The listing builds one solid part. Answer for the finished solid, in the listing's coordinates (mm). A direction names the side the tool comes from. Coordinates: 2 decimals unless noted, no trailing zeros. Write each loop counter-clockwise with the first axis right and the second up, starting at its lowest first coordinate (ties: lowest second). Pieces come first, ordered by that corner, then holes. Notation, with made-up numbers: M -26.75,-11.75 L 21.25,-11.75 A20 ccw 21.25,3.25 Z; hole C 51,66 d6. An arc over 180 degrees is marked long. Put each result on its own line as item: value. Start each with the question number.
Autodesk Inventor part; units mm, degrees
ref_plane "YZ Plane" through (0, 0, 0) normal (1, 0, 0) x (0, 1, 0)
ref_plane "XZ Plane" through (0, 0, 0) normal (0, 1, 0) x (-1, 0, 0)
ref_plane "XY Plane" through (0, 0, 0) normal (0, 0, 1) x (1, 0, 0)
sketch "Sketch1" plane through (0, 0, 0) normal (0, 1, 0) x (-1, 0, 0)
  line L0 (0, 75) -> (0, -75) construction
  arc A0 (18.258988, 69.745538) -> (-18.258988, 69.745538) centre (0, 75) ccw
  line L1 (0, -196.504208) -> (0, 248.158352) construction
  line L2 (-25.341268, -40) -> (25.341268, -40)
  line L3 (25.341268, -40) -> (20, -23.743159)
  line L4 (20, -23.743159) -> (-20, -23.743159)
  line L5 (-20, -23.743159) -> (-25.341268, -40)
  circle A1 centre (12, -31.871075) radius 2
  circle A2 centre (-12, -31.871075) radius 2
  circle A3 centre (0, -31.871075) radius 2
  circle A4 centre (0, -75) radius 23.5
  circle A5 centre (170.873428, 25.827072) radius 158.808057
  circle A6 centre (-170.873428, 25.827072) radius 158.808057
  point P0 (0, 0)
  dimension "d0" = 150
  dimension "d1" = 75
  dimension "d22" = 38
  dimension "d33" = 47
  dimension "d34" = 4
  dimension "d35" = 71.8118
  dimension "d36" = 71.8118
  dimension "d37" = 16.25684
  dimension "d38" = 35
  dimension "d39" = 35
  dimension "d40" = 0
  dimension "d41" = 48.15025
  dimension "d42" = 0
  dimension "d43" = 48.15025
  dimension "d44" = 0
  dimension "d45" = 8.12893
  dimension "d46" = 10.13733
  dimension "d47" = 8.12893
  dimension "d48" = 21.53777
  dimension "d49" = 8.12893
  dimension "d50" = 32.93821
  dimension "d51" = 0
  dimension "d52" = 16.25684
  dimension "d53" = 38.00145
  dimension "d54" = 16.25684
extrude "Extrusion1" add sketch "Sketch1" along normal blind 10 contours A5 L4 A6 A0 | L3 L2 L5 L4 | A1 | A2
sketch "Sketch4" plane through (0, 10, 0) normal (0, 1, 0) x (1, 0, 0)
  circle A0 centre (3.680608, -72.875) radius 1.5
  circle A1 centre (0, -79.25) radius 1.5
  circle A2 centre (-3.680608, -72.875) radius 1.5
  arc A3 (5.450881, -75.044363) -> (2.76386, -79.69842) centre (10.238345, -80.911111) ccw
  arc A4 (5.450881, -75.044363) -> (2.687021, -70.257217) centre (3.680608, -72.875) ccw
  arc A5 (-2.687021, -70.257217) -> (2.687021, -70.257217) centre (0, -63.177778) ccw
  arc A6 (-2.687021, -70.257217) -> (-5.450881, -75.044363) centre (-3.680608, -72.875) ccw
  arc A7 (-2.76386, -79.69842) -> (-5.450881, -75.044363) centre (-10.238345, -80.911111) ccw
  arc A8 (-2.76386, -79.69842) -> (2.76386, -79.69842) centre (0, -79.25) ccw
  point P0 (0, 0)
extrude "Extrusion4" cut sketch "Sketch4" against normal through all contours A0 | A1 | A2
sketch "Sketch5" plane through (0, 10, 0) normal (0, 1, 0) x (1, 0, 0)
  circle A0 centre (-3.680608, -72.875) radius 1.5
  circle A1 centre (-3.680608, -72.875) radius 2.225
  circle A2 centre (0, -79.25) radius 1.5
  circle A3 centre (0, -79.25) radius 2.225
  circle A4 centre (3.680608, -72.875) radius 1.5
  circle A5 centre (3.680608, -72.875) radius 2.225
  point P0 (0, 0)
  dimension "d69" = 4.45
  dimension "d70" = 4.45
  dimension "d71" = 4.45
extrude "Extrusion5" cut sketch "Sketch5" against normal blind 6 contours A0 | A1 | A2 | A3 | A4 | A5
sketch "Sketch6" plane through (0, 0, 0) normal (0, -1, 0) x (1, 0, 0)
  circle A0 centre (0, 79.25) radius 1.5
  circle A1 centre (3.680608, 72.875) radius 1.5
  circle A2 centre (-3.680608, 72.875) radius 1.5
  point P0 (0, 0)
extrude "Extrusion6" add sketch "Sketch6" against normal up to surface (4 mm away)
sketch "Sketch7" plane through (0, 0, 0) normal (0, -1, 0) x (1, 0, 0)
  circle A0 centre (23.270461, -31.871075) radius 2
  circle A1 centre (-23.270461, -31.871075) radius 2
  circle A2 centre (0, -31.871075) radius 2
  line L0 (-32.726793, -40) -> (32.726793, -40)
  line L1 (-29.32798, -23.743159) -> (29.32798, -23.743159)
  line L2 (-25.341268, -40) -> (-20, -23.743159)
  line L3 (20, -23.743159) -> (25.341268, -40)
  line L4 (29.32798, -23.743159) -> (32.726793, -40)
  line L5 (-32.726793, -40) -> (-29.32798, -23.743159)
  point P0 (0, 0)
  point P1 (22.130539, -30.227731)
  point P2 (23.327313, -33.870267)
  point P3 (-23.327313, -33.870267)
  point P4 (-22.130539, -30.227731)
extrude "Extrusion7" add sketch "Sketch7" against normal up to surface (10 mm away) contours A0 L3 | A0 L3 L1 L4 L0 | L2 A1 L0 L5 L1 | L2 A1 | A1 L2 picked at (24.149861, -31.36133)
sketch "Sketch8" plane through (0, 10, 0) normal (0, 1, 0) x (1, 0, 0)
  arc A0 (-18.258988, -69.745538) -> (18.258988, -69.745538) centre (0, -75) ccw
  line L0 (0, -75) -> (0, -57.620328) construction
  line L1 (-29.32798, 23.743159) -> (-32.726793, 40)
  line L2 (-29.32798, 23.743159) -> (-18.322098, -28.899016)
  arc A1 (-18.553855, -70.906779) -> (-18.322098, -28.899016) centre (-116.205725, -49.363513) ccw
  arc A2 (-18.258988, -69.745538) -> (18.258988, -69.745538) centre (0, -75) ccw
  circle A3 centre (0, -75) radius 19
  arc A4 (-18.258988, -69.745538) -> (-20, 23.743159) centre (-170.873428, -25.827072) ccw
  line L3 (-20, 23.743159) -> (-29.32798, 23.743159)
  arc A5 (20, 23.743159) -> (18.258988, -69.745538) centre (170.873428, -25.827072) ccw
  line L4 (29.32798, 23.743159) -> (20, 23.743159)
  line L5 (29.32798, 23.743159) -> (18.322098, -28.899016)
  arc A6 (18.322098, -28.899016) -> (18.553855, -70.906779) centre (116.205725, -49.363513) ccw
  point P0 (0, 0)
  point P1 (18.553855, -70.906779)
  point P2 (-18.553855, -70.906779)
  dimension "d80" = 100
extrude "Extrusion8" add sketch "Sketch8" against normal blind 10 contours A0 A1 L2 L3 A4 | A5 L4 L5 A6 A0
sketch "Sketch11" plane through (0, 0, 0) normal (0, -1, 0) x (1, 0, 0)
  circle A0 centre (23.270461, -31.871075) radius 2
  circle A1 centre (-23.270461, -31.871075) radius 2
  point P0 (0, 0)
extrude "Extrusion11" cut sketch "Sketch11" against normal through all
chamfer "Chamfer1" distance 2 angle 45 5 edges at (-25.5244, 0, -5.5505) (-16.2072, 0, 49.9152) (0, 0, 94) (16.2072, 0, 49.9152) (25.5244, 0, -5.5505)
sketch "Sketch17" plane through (0, 10, 0) normal (0, 1, 0) x (1, 0, 0)
  line L0 (-83.121979, 82.295999) -> (15.75457, -64.379571)
  line L1 (-29.32798, 23.743159) -> (29.32798, 23.743159)
  circle A0 centre (-23.270461, 31.871075) radius 2
  circle A1 centre (23.270461, 31.871075) radius 2
  circle A2 centre (0, 31.871075) radius 2
  arc A3 (-18.553855, -70.906779) -> (18.553855, -70.906779) centre (0, -75) ccw
  arc A4 (18.322098, -28.899016) -> (18.553855, -70.906779) centre (116.205725, -49.363513) ccw
  line L2 (32.726793, 40) -> (18.322098, -28.899016)
  line L3 (-32.726793, 40) -> (32.726793, 40)
  line L4 (-32.726793, 40) -> (-18.322098, -28.899016)
  arc A5 (-18.553855, -70.906779) -> (-18.322098, -28.899016) centre (-116.205725, -49.363513) ccw
  circle A6 centre (-3.680608, -72.875) radius 2.225
  circle A7 centre (0, -79.25) radius 2.225
  circle A8 centre (3.680608, -72.875) radius 2.225
  line L5 (15.75457, -64.379571) -> (17.86641, -67.512319)
  line L6 (-32.726793, 40) -> (-18.322098, -28.899016)
  point P0 (0, 0)
  point P1 (-22.889065, -7.054783)
extrude "Extrusion16" add sketch "Sketch17" along normal blind 9 contours L4 L1 L2 A4 L5 L0
sketch "Sketch18" plane through (0, 19, 0) normal (0, 1, 0) x (1, 0, 0)
  circle A0 centre (13.844472, -83.053003) radius 1.5
  circle A1 centre (-8.053003, -88.844472) radius 1.5
  circle A2 centre (8.053003, -61.155528) radius 1.5
  circle A3 centre (-13.844472, -66.946997) radius 1.5
  circle A4 centre (57.038778, -59.914319) radius 1.5
  circle A5 centre (0, -75) radius 12.1825
  line L0 (54.737573, -51.213489) -> (22.535282, -59.730387)
  arc A6 (59.339984, -68.61515) -> (54.737573, -51.213489) centre (57.038778, -59.914319) ccw
  line L1 (27.137693, -77.132048) -> (59.339984, -68.61515)
  arc A7 (27.137693, -77.132048) -> (15.997897, -85.250234) centre (31.995793, -95.500468) ccw
  arc A8 (8.838591, -58.180983) -> (15.997897, -85.250234) centre (0, -75) ccw
  arc A9 (8.838591, -58.180983) -> (22.535282, -59.730387) centre (17.677181, -41.361967) ccw
  arc A10 (18.322098, -28.899016) -> (17.86641, -67.512319) centre (116.205725, -49.363513) ccw
  line L2 (18.322098, -28.899016) -> (29.32798, 23.743159)
  line L3 (29.32798, 23.743159) -> (-29.32798, 23.743159)
  line L4 (-29.32798, 23.743159) -> (-22.889065, -7.054783)
  line L5 (-22.889065, -7.054783) -> (17.86641, -67.512319)
  circle A11 centre (-19.580037, -5.657222) radius 3.525
  circle A12 centre (14.082222, -57.518268) radius 2.448572
  arc A13 (18.322098, -28.899016) -> (17.86641, -67.512319) centre (116.205725, -49.363513) ccw
  point P0 (0, 0)
  point P1 (-22.502925, -7.627592)
  point P2 (-23.030435, -6.378596)
  point P3 (16.523025, -57.323365)
  point P4 (12.051896, -58.886946)
  dimension "d117" = 7.05
extrude "Extrusion17" cut sketch "Sketch18" against normal up to surface (9 mm away) contours A10 L5 A9 | A9 A12 A10 | A9 L5 A12 | L5 L4 A11
sketch "Sketch19" plane through (0, 19, 0) normal (0, 1, 0) x (1, 0, 0)
  arc A0 (-23.030435, -6.378596) -> (-22.502925, -7.627592) centre (-19.580037, -5.657222) ccw
  circle A1 centre (-19.580037, -5.657222) radius 2.225
  circle A2 centre (12.769294, -53.644906) radius 3.525 construction
  line L0 (-22.502925, -7.627592) -> (12.051896, -58.886946)
  arc A3 (18.322098, -28.899016) -> (16.523025, -57.323365) centre (116.205725, -49.363513) ccw
  circle A4 centre (12.769294, -53.644906) radius 2.225
  point P0 (0, 0)
  dimension "d120" = 4.45
  dimension "d121" = 7.05
  dimension "d122" = 4.45
extrude "Extrusion18" cut sketch "Sketch19" against normal blind 9.5
sketch "Sketch20" plane through (0, 19, 0) normal (0, 1, 0) x (1, 0, 0)
  circle A0 centre (-19.580037, -5.657222) radius 2.225
  circle A1 centre (12.769294, -53.644906) radius 2.225
  arc A2 (-23.030435, -6.378596) -> (-22.502925, -7.627592) centre (-19.580037, -5.657222) ccw
  line L0 (-22.502925, -7.627592) -> (12.051896, -58.886946)
  arc A3 (12.051896, -58.886946) -> (16.523025, -57.323365) centre (14.082222, -57.518268) ccw
  arc A4 (18.322098, -28.899016) -> (16.523025, -57.323365) centre (116.205725, -49.363513) ccw
  line L1 (18.322098, -28.899016) -> (29.32798, 23.743159)
  line L2 (29.32798, 23.743159) -> (-29.32798, 23.743159)
  line L3 (-29.32798, 23.743159) -> (-23.030435, -6.378596)
  line L4 (-13.501752, -3.090072) -> (7.292792, -33.93714)
  arc A5 (8.533736, -26.852566) -> (7.292792, -33.93714) centre (116.205725, -49.363513) ccw
  line L5 (8.533736, -26.852566) -> (17.02107, 13.743159)
  line L6 (17.02107, 13.743159) -> (-17.02107, 13.743159)
  line L7 (-17.02107, 13.743159) -> (-13.501752, -3.090072)
  point P0 (0, 0)
  dimension "d125" = 10
extrude "Extrusion19" cut sketch "Sketch20" against normal through all contours L7 L6 L5 A5 L4
fillet "Fillet2" radius 5 4 edges at (-13.5018, 9.5, 3.0901) (7.2928, 9.5, 33.9371) (-17.0211, 9.5, -13.7432) (17.0211, 9.5, -13.7432)
sketch "Sketch21" plane through (0, 10, 0) normal (0, 1, 0) x (1, 0, 0)
  line L0 (12.051896, -58.886946) -> (-22.502925, -7.627592)
  arc A0 (-23.030435, -6.378596) -> (-22.502925, -7.627592) centre (-19.580037, -5.657222) ccw
  line L1 (-23.030435, -6.378596) -> (-18.322098, -28.899016)
  arc A1 (-18.553855, -70.906779) -> (-18.322098, -28.899016) centre (-116.205725, -49.363513) ccw
  arc A2 (-18.553855, -70.906779) -> (18.553855, -70.906779) centre (0, -75) ccw
  arc A3 (16.523025, -57.323365) -> (18.553855, -70.906779) centre (116.205725, -49.363513) ccw
  arc A4 (12.051896, -58.886946) -> (16.523025, -57.323365) centre (14.082222, -57.518268) ccw
  circle A5 centre (-3.680608, -72.875) radius 2.225
  circle A6 centre (0, -79.25) radius 2.225
  circle A7 centre (3.680608, -72.875) radius 2.225
  circle A8 centre (0, -75) radius 8.5 construction
  circle A9 centre (0, -75) radius 9.35
  point P0 (0, 0)
  dimension "d129" = 17
  dimension "d130" = 0.85
extrude "Extrusion20" cut sketch "Sketch21" against normal blind 0.2 contours A4 A3 A2 A1 L1 A0 L0
chamfer "Chamfer2" distance 0.2 angle 45 1 edges at (-9.35, 9.8, 75)
properties part number "motion_thigh_bot_3DPrint"
1) Straight lines are drawn through the part: probe 1 along X at (y, z) = (12.25, 4); probe 2 along Z at (x, y) = (0, 5.65) (3 decimals); probe 3 along Y at (x, z) = (6.5, 61.5). For each, find the intervals that lie inside material, in ascending order.
2) A cutting plane is placed at A-A on x = 24. Write down the section's boundary in (y, z).
3) A cutting plane is placed at C-C on z = -22.5. Write down the section's boundary in (x, y), then the cut area to 3 significant figures.
4) A cutting plane is placed at B-B on z = 0. Write down the section's boundary in (x, y), then the cut area to 3 significant figures.
5) For faces 4 (the face through (-16.21, 5.95, 50.21)), 5 (the face through (13, 19, 8)), 6 (the face through (-4, 4, 73)), 7 (the face through (0, 10, -35)), 8 (the face through (-6.325, 9.633, 13.736)), determine the directions among +Z, -Z, +X, -X, +Y, -Y from which every point of the face is accessible in a straight line to the end or side of a thin tool.
6) Given pin 1 Ø1 at (y, z) = (10, -19.5) entering from -X; pin 2 Ø8 at (x, z) = (9.5, 2) entering from +Y; pin 3 Ø4 at (x, z) = (12.77, 53.64) entering from +Y; pin 4 Ø8 at (x, y) = (-8.5, 15) entering from -Z, each flat-ended and moving along its own axis, determine where each tip first touches the part or whether it passes through.
7) Determine the mould class of faces 1 (the face through (0, 10, 75)), 2 (the face through (0, 5, -40)), 3 (the face through (0, 10, -13.743)) for opening direction Z: +Z half, -Z half, draft (parallel to the pull), parting line (faces both ways), or undercut.
8) A cutting plane is placed at D-D on y = 15.25. State how many separate pieces and enclosed holes the cut face has, then the cut area to 3 significant figures.
Answers follow:
1. probe 1: x = -23.53 to -21.06, -18.1 to -12.89, 13.31 to 23.53
1. probe 2: z = -40 to -33.871, -29.871 to -13.743, 23.119 to 77.025, 81.475 to 94
1. probe 3: y = 0 to 9.8
2. outline: M 0,-40 L 10,-40 L 10,-33.73 L 0,-33.73 Z; M 0,-30.01 L 10,-30.01 L 10,-23.74 L 19,-23.74 L 19,1.74 L 2,1.74 L 0,-8.03 Z
3. outline: M -29.07,2 L -27.02,0 L 27.02,0 L 29.07,2 L 29.07,19 L -29.07,19 Z
3. area: 1,100 mm²
4. outline: M -24.36,2 L -22.32,0 L -14.15,0 L -14.15,19 L -24.36,19 Z; M 14.15,0 L 22.32,0 L 24.36,2 L 24.36,19 L 14.15,19 Z
4. area: 384 mm²
5. face 4: -X, +Y, -Y
5. face 5: +Z, -Z, +X, -X, +Y
5. face 6: +Y
5. face 7: -Z, +X, -X, +Y
5. face 8: +Y, -Y
6. pin 1: stops at x = -28.55
6. pin 2: passes through
6. pin 3: stops at y = 9.5
6. pin 4: stops at z = -23.74
7. face 1: draft
7. face 2: -Z half
7. face 3: undercut
8. separate pieces: 1
8. enclosed holes: 3
8. area: 1,930 mm²
